from build123d import *

# Parameters (mm, degrees)
BOSS_EXTRUDE1_DEPTH = 14
CUT_EXTRUDE1_DEPTH  = 46.814563472
CUT_EXTRUDE2_DEPTH  = 47.465040622
HOLE1_D             = 6.4
HOLE2_D             = 6.4


with BuildPart() as part:
    # Sketch1 → Boss-Extrude1 (new body)
    with BuildSketch(Plane.XY.offset(14)):
        with BuildLine():
            Line((7, 0), (7, 25.041451884))
            Line((7, 25.041451884), (6.133974596, 26.541451884))
            Line((6.133974596, 26.541451884), (-15.552558883, 39.062177826))
            ThreePointArc((-15.552558883, 39.062177826), (-25.11473671, 36.5), (-22.552558883, 26.937822174))
            Line((-22.552558883, 26.937822174), (-10.464101615, 19.958548116))
            Line((-10.464101615, 19.958548116), (-7, 13.958548116))
            Line((-7, 13.958548116), (-7, 0))
            ThreePointArc((-7, 0), (0, -7), (7, 0))
        make_face()
    extrude(amount=-BOSS_EXTRUDE1_DEPTH)

    # Sketch2 → Cut-Extrude1 (cut, through all)
    with BuildSketch(Plane(origin=(6.026279442, 10.437822174, 0), x_dir=(0.8660254037844398, -0.49999999999999806, 0), z_dir=(-0.499999999999998, -0.8660254037844397, 0))):
        with BuildLine():
            Line((-26, 11.606580927), (-28.301887361, 9.222906785))
            ThreePointArc((-28.301887361, 9.222906785), (-26, 3.8), (-23.698112639, 9.222906785))
            Line((-23.698112639, 9.222906785), (-26, 11.606580927))
        make_face()
    extrude(amount=-CUT_EXTRUDE1_DEPTH, mode=Mode.SUBTRACT)

    # Sketch3 → Cut-Extrude2 (cut, through all)
    with BuildSketch(Plane.ZY.offset(7)):
        with BuildLine():
            Line((9.222906785, 4.698112639), (11.606580927, 7))
            Line((11.606580927, 7), (9.222906785, 9.301887361))
            ThreePointArc((9.222906785, 9.301887361), (3.8, 7), (9.222906785, 4.698112639))
        make_face()
    extrude(amount=-CUT_EXTRUDE2_DEPTH, mode=Mode.SUBTRACT)

    # Hole1 (through all)
    with Locations(Plane(origin=(0, 0, 0), x_dir=(-1, 0, 0), z_dir=(0, 0, -1))):
        with Locations((0, 0)):
            Hole(HOLE1_D / 2)

    # Hole2 (through all)
    with Locations(Plane(origin=(0, 0, 0), x_dir=(-1, 0, 0), z_dir=(0, 0, -1))):
        with Locations((19.0525, 32.999898011)):
            Hole(HOLE2_D / 2)


solid = part.part
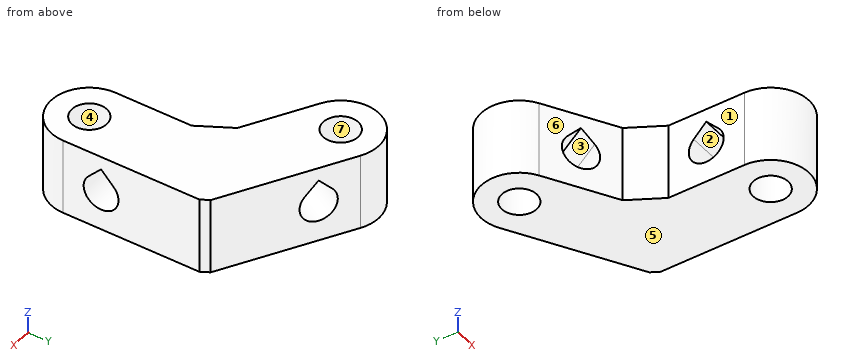
Check sheet for the modelled part. Datum: model origin and axes. Units: mm. Face numbers are marked on the shaded views. A direction names the side the tool comes from. Round coordinates to 2 decimals unless told otherwise and drop trailing zeros. Loops run counter-clockwise (first coordinate to the right, second up) from the corner with the lowest first, then second, coordinate; pieces in that order, holes last. Notation, with made-up numbers: (-4, -8) -> (1, -8) arc R15 cw to (1, 16) -> close; hole circle Ø1 at (-5.5, -39). An arc over 180 degrees is marked (long way). Put each result on its own line as item: value. Start each with the question number.
1. Scan lines: probe 1 along Y at (x, z) = (1, 8); probe 2 along X at (y, z) = (5.5, 10.25); probe 3 along Y at (x, z) = (5, 5.25). Record each from-to range of solid material in increasing order.
2. Section check D-D (y = 32). Give the number of separate pieces and of enclosed holes in the cut face, plus the area to 3 significant figures.
3. Section check A-A (x = 2). Enter the section's corners in (y, z), plus the area to 3 significant figures.
4. Section check C-C (x = -20.5). Enter the section's corners in (y, z).
5. Gauge pin test, flat ends, axial feed: pin 1 (5 mm diameter, centred on x = -22.5, z = 11, fed in from -Y); pin 2 (1 mm diameter, centred on x = -22, z = 7.5, fed in from -Y); pin 3 (4 mm diameter, centred on y = 16.5, z = 11, fed in from -X). Record the tip position at first contact, or that the pin passes through.
6. Access from +Z, -Z, +X, -X, +Y, -Y to the whole of each face (thin tool, end or side, straight path). Record for the marked faces 1, 2 and 3.
7. Section check B-B (z = 7.25). Enter the section's corners in (x, y), plus the area to 3 significant figures.
8. Draft check along Y on the marked faces 4, 5, 6 and 7. Enter one of: +Y half, -Y half, draft (parallel to the pull), parting line (faces both ways), or undercut.
Findings:
1. probe 1: y = -6.93 to -3.04, 3.04 to 3.96, 10.04 to 29.51
1. probe 2: x = -7 to 7
1. probe 3: y = -4.9 to 4.32, 9.68 to 27.2
2. separate pieces: 2
2. enclosed holes: 1
2. area: 192 mm^2
3. outline: (-6.71, 0) -> (-2.5, 0) -> (-2.5, 14) -> (-6.71, 14) -> close; (2.5, 0) -> (28.93, 0) -> (28.93, 14) -> (2.5, 14) -> close; hole (4.7, 9.22) arc R3.2 ccw (long way) to (9.3, 9.22) -> (7, 11.61) -> close
3. area: 394 mm^2
4. outline: (25.75, 0) -> (30.15, 0) -> (30.15, 14) -> (25.75, 14) -> close; (35.85, 0) -> (39.85, 0) -> (39.85, 14) -> (35.85, 14) -> close
5. pin 1: stops at y = 25.46
5. pin 2: stops at y = 26.33
5. pin 3: stops at x = -9.62
6. face 1: +Z, -Z, -X, -Y
6. face 2: +X, -X
6. face 3: none
7. outline: (-22.55, 26.94) -> (-19.25, 25.03) -> (-12.25, 37.16) -> (-15.55, 39.06) arc R7 ccw to start; (-13.73, 21.84) -> (-10.46, 19.96) -> (-7, 13.96) -> (-7, 10.19) -> (7, 10.19) -> (7, 25.04) -> (6.13, 26.54) -> (-6.73, 33.97) -> close; (-7, 0) arc R7 ccw to (7, 0) -> (7, 3.81) -> (-7, 3.81) -> close; hole circle Ø6.4 at (-19.05, 33); hole circle Ø6.4 at (0, 0)
7. area: 533 mm^2
8. face 4: undercut
8. face 5: draft
8. face 6: -Y half
8. face 7: undercut
